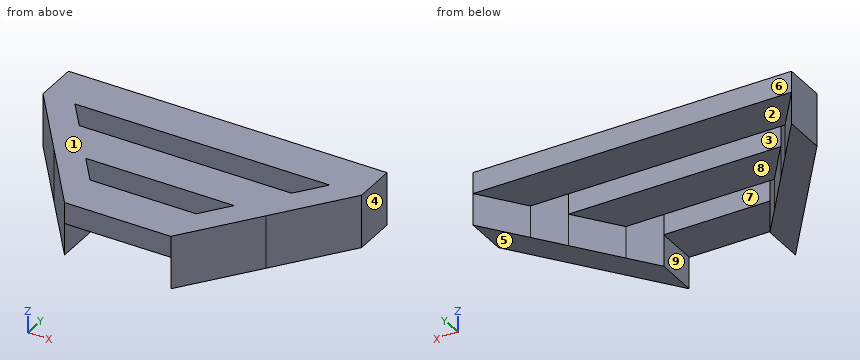
```python
from build123d import *

# Parameters (mm, degrees)
F1_DEPTH = 5
F2_START = 3
F0_W     = 10
F0_H     = 4
F2_DEPTH = 2


with BuildPart() as f1:
    # F0 (on Top) → F1 (new body)
    with BuildSketch(Plane.XY):
        Polygon((-15, 21.9410226196), (-15, 17.9410226196), (-11.9911272283, 17.9410226196), align=None)
        Polygon((-11.9911272283, 17.9410226196), (-15, 17.9410226196), (-10, 11.2940150797), (-10, 15.2940150797), align=None)
        Polygon((-10, 15.2940150797), (-10, 11.2940150797), (-6.9911272283, 11.2940150797), align=None)
        Polygon((-6.9911272283, 11.2940150797), (-10, 11.2940150797), (-5, 4.6470075399), (-5, 8.6470075399), align=None)
    extrude(amount=F1_DEPTH)



with BuildPart() as f1b:
    # F0 (on Top) → F1, piece 2 (new body)
    with BuildSketch(Plane.XY):
        Polygon((10, 11.2940150797), (6.9911272283, 11.2940150797), (5, 8.6470075399), (5, 4.6470075399), align=None)
        Polygon((10, 11.2940150797), (10, 15.2940150797), (6.9911272283, 11.2940150797), align=None)
        Polygon((15, 17.9410226196), (11.9911272283, 17.9410226196), (10, 15.2940150797), (10, 11.2940150797), align=None)
        Polygon((15, 21.9410226196), (11.9911272283, 17.9410226196), (15, 17.9410226196), align=None)
    extrude(amount=F1_DEPTH)


with BuildPart() as f1_1:
    add(f1.part)

    add(f1b.part)  # F2 merges F1b
    # F0 (on Top) → F2 (join)
    with BuildSketch(Plane.XY.offset(F2_START)):
        with Locations((0, 6.6470075399)):
            Rectangle(F0_W, F0_H)
        Polygon((10, 15.2940150797), (-10, 15.2940150797), (-6.9911272283, 11.2940150797), (6.9911272283, 11.2940150797), align=None)
        Polygon((-15, 21.9410226196), (-11.9911272283, 17.9410226196), (11.9911272283, 17.9410226196), (15, 21.9410226196), align=None)
    extrude(amount=F2_DEPTH)


solid = f1_1.part
```
Geometry check sheet. Reference: the model listing, model coordinates, mm. Face numbers are marked on the shaded views. A direction names the side the tool comes from. Coordinates: 2 decimals unless noted, no trailing zeros. Order: outer loops, then holes, each group sorted by start corner. A loop starts at its lowest first (then second) coordinate and runs counter-clockwise, first axis right, second up. Notation, with made-up numbers: (36.5, 51.25) - (58.5, 51.25) arc R12 ccw to (58.5, 72.25) - close; hole circle Ø5 at (67.5, 29.5). An arc over 180 degrees is marked (long way). Use one line per item in the form item = value.
1. Section check A-A (x = 1.5). Record the boundary of the cut face in (y, z), then the cut area to 3 significant figures.
Here are the results:
outline = (4.65, 3) - (8.65, 3) - (8.65, 5) - (4.65, 5) - close; (11.29, 3) - (15.29, 3) - (15.29, 5) - (11.29, 5) - close; (17.94, 3) - (21.94, 3) - (21.94, 5) - (17.94, 5) - close
area = 24.0 mm²
2. Section check D-D (z = 4). Record the boundary of the cut face in (x, y).
Here are the results:
outline = (-15, 17.94) - (-5, 4.65) - (5, 4.65) - (15, 17.94) - (15, 21.94) - (-15, 21.94) - close; hole (-11.99, 17.94) - (-10, 15.29) - (10, 15.29) - (11.99, 17.94) - close; hole (-6.99, 11.29) - (-5, 8.65) - (5, 8.65) - (6.99, 11.29) - close
3. Section check C-C (y = 9.5). Record the boundary of the cut face in (x, z), then the cut area to 3 significant figures.
Here are the results:
outline = (-8.65, 0) - (-5.64, 0) - (-5.64, 5) - (-8.65, 5) - close; (5.64, 0) - (8.65, 0) - (8.65, 5) - (5.64, 5) - close
area = 30.1 mm²
4. Scan lines: line 1 (Y direction, x = -1.75, z = 3.15); line 2 (Z direction, x = 1.25, y = 6.5); line 3 (Y direction, x = -6.25, z = 3.5). Record each from-to range of solid material in increasing order.
Here are the results:
line_1 = 4.65 to 8.65, 11.29 to 15.29, 17.94 to 21.94
line_2 = 3 to 5
line_3 = 6.31 to 10.31, 11.29 to 15.29, 17.94 to 21.94
5. Gauge pin test, flat ends, axial feed: pin 1 (1.5 mm diameter, centred on y = 13, z = 1, fed in from +X); pin 2 (4 mm diameter, centred on x = 0.5, y = 11.5, fed in from -Z); pin 3 (1 mm diameter, centred on x = -4.5, y = 17, fed in from -Z); pin 4 (2 mm diameter, centred on y = 10.5, z = 3.5, fed in from -X). Record the tip position at first contact, or that the pin passes through.
Here are the results:
pin_1 = 11.85
pin_2 = 3
pin_3 = through
pin_4 = -10.15
6. Section check B-B (z = 0.95). Record the boundary of the cut face in (x, y).
Here are the results:
outline = (-15, 17.94) - (-5, 4.65) - (-5, 8.65) - (-15, 21.94) - close; (5, 4.65) - (15, 17.94) - (15, 21.94) - (5, 8.65) - close
7. Access from +Z, -Z, +X, -X, +Y, -Y to the whole of each face (thin tool, end or side, straight path). Record for the marked faces 5, 6, 7, 8 and 9.
Here are the results:
face_5 = -Z, +X, -X, +Y, -Y
face_6 = +Z, -Z, +X, -X, +Y
face_7 = +Z, -Z
face_8 = -Z, +Y
face_9 = -Z, +Y, -Y
8. Draft check along X on the marked faces 1, 2, 3 and 4. Enter one of: pulls with the +X half, pulls with the -X half, needs draft (parallel to the pull), parting line crosses it, or undercut.
Here are the results:
face_1 = needs draft
face_2 = undercut
face_3 = undercut
face_4 = pulls with the +X half
